Autodesk Inventor part; units mm, degrees
ref_plane "YZ Plane" through (0, 0, 0) normal (1, 0, 0) x (0, 1, 0)
ref_plane "XZ Plane" through (0, 0, 0) normal (0, 1, 0) x (-1, 0, 0)
ref_plane "XY Plane" through (0, 0, 0) normal (0, 0, 1) x (1, 0, 0)
sketch "Sketch1" plane through (0, 0, 0) normal (0, 0, 1) x (1, 0, 0)
  line L0 (0, 0) -> (41.5, 0)
  line L1 (41.5, 0) -> (41.5, -73)
  line L2 (41.5, -73) -> (0, -73)
  line L3 (0, -73) -> (0, 0)
  line L4 (0, -73) -> (3.11, -73)
  line L5 (0, -73) -> (3.11, -73) construction
  line L6 (3.11, -73) -> (3.11, -69.85)
  line L7 (3.11, -73) -> (6.26, -73) construction
  line L8 (3.11, -69.85) -> (14.54, -69.85)
  line L9 (14.54, -69.85) -> (19.65, -69.85)
  line L10 (19.65, -69.85) -> (31.08, -69.85)
  circle A0 centre (3.11, -69.85) radius 1.6
  circle A1 centre (14.54, -69.85) radius 1.6
  circle A2 centre (19.65, -69.85) radius 1.6
  circle A3 centre (31.08, -69.85) radius 1.6
  line L11 (3.11, -69.85) -> (3.11, -55.42)
  line L12 (3.11, -69.85) -> (17.54, -69.85) construction
  line L13 (0, -73) -> (4.33, -73)
  line L14 (0, -73) -> (4.33, -73) construction
  line L15 (4.33, -73) -> (4.33, -53.49)
  line L16 (3.11, -55.42) -> (6.6479, -55.42)
  circle A4 centre (4.33, -55.42) radius 1.651
  line L17 (4.33, -55.42) -> (4.33, -37.69)
  line L18 (4.33, -55.42) -> (22.06, -55.42) construction
  line L19 (4.33, -55.42) -> (29.68, -55.42)
  line L20 (4.33, -55.42) -> (29.68, -55.42) construction
  circle A5 centre (4.33, -37.69) radius 1.651
  circle A6 centre (29.68, -55.42) radius 1.651
  line L21 (4.33, -37.69) -> (39.0376, -37.69)
  line L22 (29.68, -55.42) -> (29.68, -25.3245)
  circle A7 centre (29.68, -37.69) radius 1.651
  line L23 (4.33, -37.69) -> (4.33, -30.44)
  line L24 (4.33, -37.69) -> (11.58, -37.69) construction
  line L25 (4.33, -30.44) -> (4.33, -12.71)
  line L26 (4.33, -30.44) -> (29.68, -30.44)
  line L27 (4.33, -30.44) -> (29.68, -30.44) construction
  line L28 (4.33, -12.71) -> (29.68, -12.71)
  circle A8 centre (29.48, -12.71) radius 1.651
  circle A9 centre (4.33, -12.71) radius 1.651
  circle A10 centre (4.33, -30.44) radius 1.651
  circle A11 centre (29.68, -30.44) radius 1.651
  dimension "d0" = 41.5
  dimension "d1" = 73
  dimension "d2" = 3.11
  dimension "d3" = 0
  dimension "d4" = 3.15
  dimension "d5" = 90
  dimension "d6" = 11.43
  dimension "d7" = 90
  dimension "d9" = 5.11
  dimension "d10" = 11.43
  dimension "d11" = 180
  dimension "d12" = 3.2
  dimension "d13" = 3.2
  dimension "d14" = 3.2
  dimension "d15" = 3.2
  dimension "d18" = 14.43
  dimension "d19" = 90
  dimension "d20" = 4.33
  dimension "d21" = 0
  dimension "d22" = 3.302
  dimension "d23" = 17.73
  dimension "d24" = 90
  dimension "d25" = 25.35
  dimension "d26" = 0
  dimension "d27" = 3.302
  dimension "d28" = 3.302
  dimension "d29" = 3.302
  dimension "d30" = 7.25
  dimension "d31" = 90
  dimension "d32" = 17.73
  dimension "d33" = 180
  dimension "d34" = 25.35
  dimension "d35" = 0
  dimension "d36" = 25.35
  dimension "d37" = 3.302
  dimension "d38" = 3.302
  dimension "d39" = 3.302
  dimension "d40" = 3.302
extrude "Extrusion2" add sketch "Sketch1" along normal blind 2 contours L0 L1 L2 L15 A0 A4 L16 L19 A6 L22 A7 A11 L26 A10 L23 A5 L17 L11 L6 L3 | L6 A0 L15 L2 | L11 A4 L15 A0 | L15 L17 A5 L21 A7 L22 A6 L19 L16 A4 | L23 A10 L26 A11 L22 A7 L21 A5
properties part number "mountPCB"
Input: part model. Units: mm. Frame: model coordinates. Coordinates: 2 decimals unless noted, no trailing zeros. Loops run counter-clockwise (first coordinate to the right, second up) from the corner with the lowest first, then second, coordinate; pieces in that order, holes last.
(1) Section C-C on y = -69.85. Return the cut outline in (x, z), then the cut area to 3 significant figures.
(2) Material intervals for probe 1 along X at (y, z) = (-30.44, 1.35); probe 2 along X at (y, z) = (-69.85, 1.4); probe 3 along Y at (x, z) = (19.5, 0.5), sorted ascending.
(3) Pull-direction query (X, two-part tool) for faces 1 (the face through (41.5, -36, 1)), 2 (the face through (30.73, -68.29, 0.99)), 3 (the face through (20, 0, 1)); classes: released by +X, released by -X, zero draft, split by the parting line, or undercut.
(4) Section B-B on z = 1. Count the separate pieces of the cut face and the enclosed holes in it, then the cut area to 3 significant figures.
(5) First-contact query: pin 1 Ø5.5 at (x, y) = (4.33, -12.71) entering from +Z. Flat tip, straight axial feed; report the tip coordinate or a pass-through.
(6) Section A-A on y = -55.42. Return the cut outline in (x, z).
(7) Section D-D on x = 14.54. Return the cut outline in (y, z).
Data:
1. outline: (0, 0) - (1.51, 0) - (1.51, 2) - (0, 2) - close; (4.71, 0) - (12.94, 0) - (12.94, 2) - (4.71, 2) - close; (16.14, 0) - (18.05, 0) - (18.05, 2) - (16.14, 2) - close; (21.25, 0) - (29.48, 0) - (29.48, 2) - (21.25, 2) - close; (32.68, 0) - (41.5, 0) - (41.5, 2) - (32.68, 2) - close
1. area: 57.4 mm2
2. probe 1: x = 0 to 2.68, 5.98 to 28.03, 31.33 to 41.5
2. probe 2: x = 0 to 1.51, 4.71 to 12.94, 16.14 to 18.05, 21.25 to 29.48, 32.68 to 41.5
2. probe 3: y = -73 to -71.44, -68.26 to 0
3. face 1: released by +X
3. face 2: undercut
3. face 3: zero draft
4. separate pieces: 1
4. enclosed holes: 12
4. area: 2,930 mm2
5. pin 1: stops at z = 2
6. outline: (0, 0) - (2.68, 0) - (2.68, 2) - (0, 2) - close; (5.98, 0) - (28.03, 0) - (28.03, 2) - (5.98, 2) - close; (31.33, 0) - (41.5, 0) - (41.5, 2) - (31.33, 2) - close
7. outline: (-73, 0) - (-71.45, 0) - (-71.45, 2) - (-73, 2) - close; (-68.25, 0) - (0, 0) - (0, 2) - (-68.25, 2) - close
